Source: CAD feature listing. Evaluate the final solid. Frame: model axes, mm. Face numbers are marked on the shaded views. A direction names the side the tool comes from. Give positions to 0.01 mm unless a question says otherwise; leave off trailing zeros. Order: outer loops, then holes, each group sorted by start corner. A loop starts at its lowest first (then second) coordinate and runs counter-clockwise, first axis right, second up. Notation, with made-up numbers: M 27,84 L 40,84 A23 ccw 40,102 Z; hole C -24.5,-23 d10. An arc over 180 degrees is marked long. Use CSV: the item, a comma, the result in double quotes. Start each with the question number.
Item 1: Pull-direction query (Y, two-part tool) for the marked faces 1, 2 and 3; classes: +Y half, -Y half, draft (parallel to the pull), parting line (faces both ways), or undercut.
Item 2: Section query A-A on z = 0.75. Count the separate pieces of the cut face and the enclosed holes in it, and give its area (3 significant figures).
Item 3: First-contact query: pin 1 (2 mm diameter, centred on y = 6, z = 0, fed in from +X); pin 2 (1.8 mm diameter, centred on x = 0.5, y = 1, fed in from -Z); pin 3 (1 mm diameter, centred on x = -3.5, y = 5.5, fed in from +Z). Flat tips, straight axial feed; report the tip coordinate or a pass-through.
Item 4: Access query for the marked faces 4, 5 and 6. Directions: +Z, -Z, +X, -X, +Y, -Y. A direction counts if a zero-diameter tool reaches every point of the face in a straight line with its end or side. Return the directions, or none.
Item 5: Ray query, probe 1 along Z at (x, y) = (6.25, -1); probe 2 along Y at (x, z) = (6.5, 0.4); probe 3 along X at (y, z) = (1, -0.3). Return the intervals inside material, ascending. Write a range as from..to.
Item 6: Section query C-C on z = 3.75. Return loops of the section in (x, y).
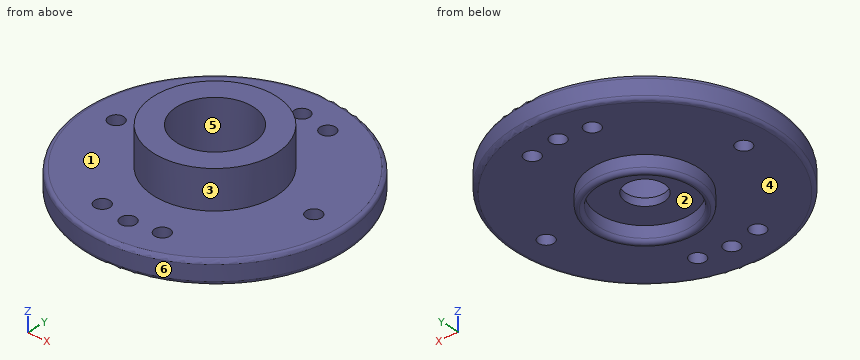
from build123d import *

# Parameters (mm, degrees)
SKETCH1_R           = 8.5
SKETCH1_R_2         = 4
SKETCH1_R_3         = 0.5
SKETCH1_R_4         = 3.5
SKETCH1_R_5         = 3
SKETCH1_R_6         = 2.5
SKETCH1_R_7         = 1.25
BOSS_EXTRUDE1_DEPTH = 0.5
SKETCH1_4_R         = 8.5
SKETCH1_4_R_2       = 4
SKETCH1_4_R_3       = 0.5
SKETCH1_4_R_4       = 3.5
SKETCH1_4_R_5       = 3
SKETCH1_4_R_6       = 2.5
BOSS_EXTRUDE2_DEPTH = 1.5
SKETCH1_5_R         = 4
SKETCH1_5_R_2       = 3.5
SKETCH1_5_R_3       = 3
SKETCH1_5_R_4       = 2.5
BOSS_EXTRUDE3_DEPTH = 4
SKETCH1_6_R         = 3.5
SKETCH1_6_R_2       = 3
BOSS_EXTRUDE4_DEPTH = 1
FILLET1_R           = 0.25


with BuildPart() as part:
    # Sketch1 → Boss-Extrude1 (new body)
    # profile 1 of 5: a face of its own
    with BuildSketch(Plane.XY):
        Circle(SKETCH1_R)
        Circle(SKETCH1_R_2, mode=Mode.SUBTRACT)
        with Locations((1.976189627, -6.192307692)):
            Circle(SKETCH1_R_3, mode=Mode.SUBTRACT)
        with Locations((-1.976189627, -6.192307692)):
            Circle(SKETCH1_R_3, mode=Mode.SUBTRACT)
        with Locations((1.976189627, 6.192307692)):
            Circle(SKETCH1_R_3, mode=Mode.SUBTRACT)
        with Locations((-1.976189627, 6.192307692)):
            Circle(SKETCH1_R_3, mode=Mode.SUBTRACT)
        with Locations((6.5, 0)):
            Circle(SKETCH1_R_3, mode=Mode.SUBTRACT)
        with Locations((-6.5, 0)):
            Circle(SKETCH1_R_3, mode=Mode.SUBTRACT)
        with Locations((0, -6.5)):
            Circle(SKETCH1_R_3, mode=Mode.SUBTRACT)
        with Locations((0, 6.5)):
            Circle(SKETCH1_R_3, mode=Mode.SUBTRACT)
    # profile 2 of 5: a face of its own
    with BuildSketch(Plane.XY):
        Circle(SKETCH1_R_2)
        Circle(SKETCH1_R_4, mode=Mode.SUBTRACT)
    # profile 3 of 5: a face of its own
    with BuildSketch(Plane.XY):
        Circle(SKETCH1_R_4)
        Circle(SKETCH1_R_5, mode=Mode.SUBTRACT)
    # profile 4 of 5: a face of its own
    with BuildSketch(Plane.XY):
        Circle(SKETCH1_R_5)
        Circle(SKETCH1_R_6, mode=Mode.SUBTRACT)
    # profile 5 of 5: a face of its own
    with BuildSketch(Plane.XY):
        Circle(SKETCH1_R_6)
        Circle(SKETCH1_R_7, mode=Mode.SUBTRACT)
    extrude(amount=BOSS_EXTRUDE1_DEPTH)

    # Sketch1<4> → Boss-Extrude2 (add)
    # profile 1 of 4: a face of its own
    with BuildSketch(Plane.XY):
        Circle(SKETCH1_4_R)
        Circle(SKETCH1_4_R_2, mode=Mode.SUBTRACT)
        with Locations((1.976189627, -6.192307692)):
            Circle(SKETCH1_4_R_3, mode=Mode.SUBTRACT)
        with Locations((-1.976189627, -6.192307692)):
            Circle(SKETCH1_4_R_3, mode=Mode.SUBTRACT)
        with Locations((1.976189627, 6.192307692)):
            Circle(SKETCH1_4_R_3, mode=Mode.SUBTRACT)
        with Locations((-1.976189627, 6.192307692)):
            Circle(SKETCH1_4_R_3, mode=Mode.SUBTRACT)
        with Locations((6.5, 0)):
            Circle(SKETCH1_4_R_3, mode=Mode.SUBTRACT)
        with Locations((-6.5, 0)):
            Circle(SKETCH1_4_R_3, mode=Mode.SUBTRACT)
        with Locations((0, -6.5)):
            Circle(SKETCH1_4_R_3, mode=Mode.SUBTRACT)
        with Locations((0, 6.5)):
            Circle(SKETCH1_4_R_3, mode=Mode.SUBTRACT)
    # profile 2 of 4: a face of its own
    with BuildSketch(Plane.XY):
        Circle(SKETCH1_4_R_2)
        Circle(SKETCH1_4_R_4, mode=Mode.SUBTRACT)
    # profile 3 of 4: a face of its own
    with BuildSketch(Plane.XY):
        Circle(SKETCH1_4_R_4)
        Circle(SKETCH1_4_R_5, mode=Mode.SUBTRACT)
    # profile 4 of 4: a face of its own
    with BuildSketch(Plane.XY):
        Circle(SKETCH1_4_R_5)
        Circle(SKETCH1_4_R_6, mode=Mode.SUBTRACT)
    extrude(amount=BOSS_EXTRUDE2_DEPTH)

    # Sketch1<5> → Boss-Extrude3 (add)
    # profile 1 of 3: a face of its own
    with BuildSketch(Plane.XY):
        Circle(SKETCH1_5_R)
        Circle(SKETCH1_5_R_2, mode=Mode.SUBTRACT)
    # profile 2 of 3: a face of its own
    with BuildSketch(Plane.XY):
        Circle(SKETCH1_5_R_2)
        Circle(SKETCH1_5_R_3, mode=Mode.SUBTRACT)
    # profile 3 of 3: a face of its own
    with BuildSketch(Plane.XY):
        Circle(SKETCH1_5_R_3)
        Circle(SKETCH1_5_R_4, mode=Mode.SUBTRACT)
    extrude(amount=BOSS_EXTRUDE3_DEPTH)

    # Sketch1<6> → Boss-Extrude4 (add)
    with BuildSketch(Plane.XY):
        Circle(SKETCH1_6_R)
        Circle(SKETCH1_6_R_2, mode=Mode.SUBTRACT)
    extrude(amount=-BOSS_EXTRUDE4_DEPTH)

    # Fillet1
    fillet1_edges = [part.edges().sort_by_distance(p)[0] for p in [
        (-8.5, 0, 0),
        (-8.5, 0, 1.5),
        (-3.5, 0, -1),
        (-3, 0, -1),
    ]]
    fillet(fillet1_edges, radius=FILLET1_R - 0.0001)  # a hair under: the kernel refuses the full size


solid = part.part
Verdict:
1,face 1,"draft"
1,face 2,"undercut"
1,face 3,"parting line"
2,separate pieces,"1"
2,enclosed holes,"9"
2,area,"201 mm2"
3,pin 1,"x = 6.85"
3,pin 2,"z = 0"
3,pin 3,"z = 1.5"
4,face 4,"-Z"
4,face 5,"+Z"
4,face 6,"+Z, -Z"
5,probe 1,"0..1.5"
5,probe 2,"-5.48..-0.5, 0.5..5.48"
5,probe 3,"-3.35..-2.83, 2.83..3.35"
6,outline,"C 0,0 d8; hole C 0,0 d5"
